Autodesk Inventor part; units mm, degrees
ref_plane "YZ Plane" through (0, 0, 0) normal (1, 0, 0) x (0, 1, 0)
ref_plane "XZ Plane" through (0, 0, 0) normal (0, 1, 0) x (-1, 0, 0)
ref_plane "XY Plane" through (0, 0, 0) normal (0, 0, 1) x (1, 0, 0)
sketch "Sketch1" plane through (0, 0, 0) normal (0, 1, 0) x (-1, 0, 0)
  line L0 (0, 0) -> (0, -48.84)
  line L1 (0, -48.84) -> (30, -48.84)
  line L2 (30, -48.84) -> (30, 0)
  line L3 (30, 0) -> (0, 0)
  circle A0 centre (4.5, -44.42) radius 1.6
  circle A1 centre (25.5, -44.42) radius 1.6
  circle A2 centre (15, -24.42) radius 6.25
  circle A3 centre (6.5, -32.92) radius 1.6
  circle A4 centre (23.5, -32.92) radius 1.6
  circle A5 centre (6.5, -15.92) radius 1.6
  circle A6 centre (23.5, -15.92) radius 1.6
  circle A7 centre (4.5, -4.42) radius 1.6
  circle A8 centre (25.5, -4.42) radius 1.6
  line L4 (23.5, -32.92) -> (23.5, -15.92)
  line L5 (23.5, -24.42) -> (6.5, -24.42)
  line L6 (25.5, -44.42) -> (4.5, -44.42)
  line L7 (4.5, -44.42) -> (4.5, -4.42)
  point P0 (30, -24.42)
  point P1 (15, -48.84)
  point P2 (15, -24.42)
  point P3 (4.5, -24.42)
  point P4 (0, -24.42)
  point P5 (15, -44.42)
  dimension "d0" = 48.84
  dimension "d1" = 30
  dimension "d2" = 12.5
  dimension "d3" = 17
  dimension "d4" = 17
  dimension "d5" = 3.2
  dimension "d6" = 21
  dimension "d7" = 40
extrude "Extrusion1" add sketch "Sketch1" along normal blind 5
sketch "Sketch2" plane through (0, 0, 0) normal (0, -1, 0) x (1, 0, 0)
  circle A0 centre (-23.5, -15.92) radius 1.6 construction
  circle A1 centre (-4.5, -4.42) radius 1.6 construction
  circle A2 centre (-25.5, -44.42) radius 1.6 construction
  circle A3 centre (-25.5, -4.42) radius 1.6 construction
  circle A4 centre (-4.5, -44.42) radius 1.6 construction
  circle A5 centre (-6.5, -32.92) radius 1.6 construction
  circle A6 centre (-23.5, -32.92) radius 1.6 construction
  circle A7 centre (-6.5, -15.92) radius 1.6 construction
  circle A8 centre (-4.5, -44.42) radius 1.6
  circle A9 centre (-6.5, -32.92) radius 1.6
  circle A10 centre (-6.5, -15.92) radius 1.6
  circle A11 centre (-4.5, -4.42) radius 1.6
  circle A12 centre (-25.5, -4.42) radius 1.6
  circle A13 centre (-23.5, -15.92) radius 1.6
  circle A14 centre (-23.5, -32.92) radius 1.6
  circle A15 centre (-25.5, -44.42) radius 1.6
extrude "Extrusion2" add sketch "Sketch2" against normal blind 17.5
properties part number "Plate"
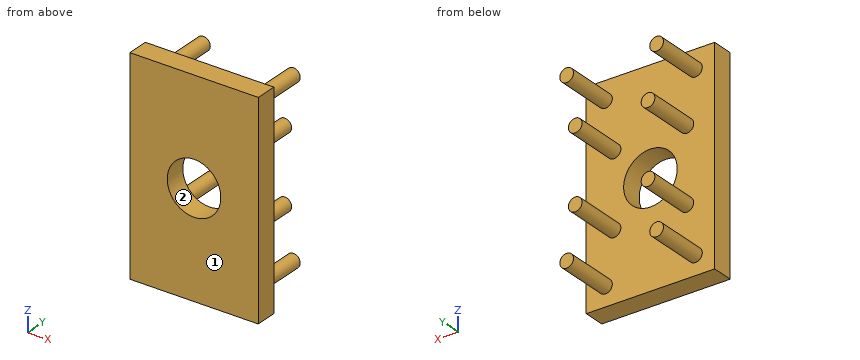
Source: CAD feature listing. Evaluate the final solid. Frame: model axes, mm. Face numbers are marked on the shaded views. Round coordinates to 2 decimals unless told otherwise and drop trailing zeros. Loops run counter-clockwise (first coordinate to the right, second up) from the corner with the lowest first, then second, coordinate; pieces in that order, holes last.
1. Section query B-B on x = -13. Output: boundary loops of the cut face in (y, z).
2. Section query C-C on z = -32.92. Output: boundary loops of the cut face in (x, y), and give its area (3 significant figures).
3. Ray query, L1, parallel to Z at x = -15, y = 1.4; L2, parallel to X at y = 1.25, z = -24.42; L3, parallel to Y at x = -17, z = -33.5. Return the intervals inside material, ascending.
4. Section query D-D on z = -19. Output: boundary loops of the cut face in (x, y).
5. Mould query, pull axis X, two halves, no side actions, for the marked faces 1 and 2. Classes: released by +X, released by -X, zero draft, split by the parting line, or undercut.
6. Section query A-A on y = 11. Output: boundary loops of the cut face in (x, z).
7. Contact query for flat-ended pins moving along their axis: pin 1 (2 mm diameter, centred on x = -7.5, y = 9, fed in from -Z); pin 2 (4 mm diameter, centred on x = -4.5, z = -13.5, fed in from -Y); pin 3 (4 mm diameter, centred on x = -12, z = -21, fed in from +Y). Output: stop coordinate, or through.
Answers below:
1. outline: (0, -48.84) - (5, -48.84) - (5, -30.34) - (0, -30.34) - close; (0, -18.5) - (5, -18.5) - (5, 0) - (0, 0) - close
2. outline: (-30, 0) - (0, 0) - (0, 5) - (-4.9, 5) - (-4.9, 17.5) - (-8.1, 17.5) - (-8.1, 5) - (-21.9, 5) - (-21.9, 17.5) - (-25.1, 17.5) - (-25.1, 5) - (-30, 5) - close
2. area: 230 mm2
3. L1: z = -48.84 to -30.67, -18.17 to 0
3. L2: x = -30 to -21.25, -8.75 to 0
3. L3: y = 0 to 5
4. outline: (-30, 0) - (-18.11, 0) - (-18.11, 5) - (-30, 5) - close; (-11.89, 0) - (0, 0) - (0, 5) - (-11.89, 5) - close
5. face 1: zero draft
5. face 2: undercut
6. outline: circle Ø3.2 at (-25.5, -44.42); circle Ø3.2 at (-25.5, -4.42); circle Ø3.2 at (-23.5, -32.92); circle Ø3.2 at (-23.5, -15.92); circle Ø3.2 at (-6.5, -32.92); circle Ø3.2 at (-6.5, -15.92); circle Ø3.2 at (-4.5, -44.42); circle Ø3.2 at (-4.5, -4.42)
7. pin 1: stops at z = -34.52
7. pin 2: stops at y = 0
7. pin 3: stops at y = 5
